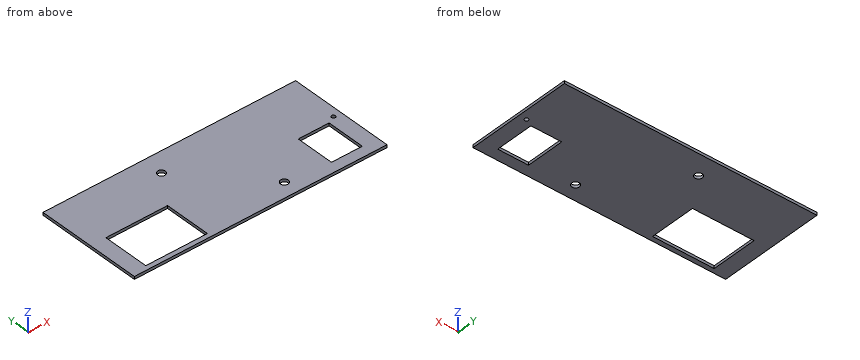
```python
from build123d import *

# Parameters (mm, degrees)
SKETCH_W      = 164
SKETCH_H      = 68.8
PAD_DEPTH     = 1.8
SKETCH001_R   = 2.5
SKETCH001_R_2 = 1.25
SKETCH001_W   = 40
SKETCH001_H   = 30
SKETCH001_W_2 = 20
SKETCH001_H_2 = 25
POCKET_DEPTH  = 5


with BuildPart() as part:
    # Sketch → Pad (new body)
    with BuildSketch(Plane.XY):
        with Locations((82, 34.4)):
            Rectangle(SKETCH_W, SKETCH_H)
    extrude(amount=PAD_DEPTH)

    # Sketch001 (on Face6 of Pad) → Pocket (cut)
    with BuildSketch(Plane.XY.offset(1.8)):
        with Locations((65, 55)):
            Circle(SKETCH001_R)
        with Locations((106, 10)):
            Circle(SKETCH001_R)
        with Locations((159, 34.5)):
            Circle(SKETCH001_R_2)
        with Locations((30, 18)):
            Rectangle(SKETCH001_W, SKETCH001_H)
        with Locations((144, 19.5)):
            Rectangle(SKETCH001_W_2, SKETCH001_H_2)
    extrude(amount=-POCKET_DEPTH, mode=Mode.SUBTRACT)


solid = part.part
```
Work out the finished part from the listing and answer in its coordinate system (mm). Give positions to 0.01 mm unless a question says otherwise; leave off trailing zeros. Order: outer loops, then holes, each group sorted by start corner. A loop starts at its lowest first (then second) coordinate and runs counter-clockwise, first axis right, second up.
1. Section C-C, the plane y = 55 is taken. Determine the outline of the cut face in (x, z).
Result sheet:
outline: (0, 0) - (62.5, 0) - (62.5, 1.8) - (0, 1.8) - close; (67.5, 0) - (164, 0) - (164, 1.8) - (67.5, 1.8) - close
2. Section B-B, the plane x = 142 is taken. Determine the outline of the cut face in (y, z), and give its area (3 significant figures).
Result sheet:
outline: (0, 0) - (7, 0) - (7, 1.8) - (0, 1.8) - close; (32, 0) - (68.8, 0) - (68.8, 1.8) - (32, 1.8) - close
area: 78.8 mm2
3. Section D-D, the plane z = 0.4 is taken. Determine the outline of the cut face in (x, y), and give its area (3 significant figures).
Result sheet:
outline: (0, 0) - (164, 0) - (164, 68.8) - (0, 68.8) - close; hole (10, 3) - (50, 3) - (50, 33) - (10, 33) - close; hole circle Ø5 at (65, 55); hole circle Ø5 at (106, 10); hole (134, 7) - (154, 7) - (154, 32) - (134, 32) - close; hole circle Ø2.5 at (159, 34.5)
area: 9,540 mm2
4. Section A-A, the plane y = 10 is taken. Determine the outline of the cut face in (x, z).
Result sheet:
outline: (0, 0) - (10, 0) - (10, 1.8) - (0, 1.8) - close; (50, 0) - (103.5, 0) - (103.5, 1.8) - (50, 1.8) - close; (108.5, 0) - (134, 0) - (134, 1.8) - (108.5, 1.8) - close; (154, 0) - (164, 0) - (164, 1.8) - (154, 1.8) - close
5. Straight lines are drawn through the part: L1, parallel to X at y = 28.5, z = 0.65; L2, parallel to Y at x = 106, z = 0.4; L3, parallel to Y at x = 159, z = 1.25. For each, find the intervals that lie inside material, in ascending order.
Result sheet:
L1: x = 0 to 10, 50 to 134, 154 to 164
L2: y = 0 to 7.5, 12.5 to 68.8
L3: y = 0 to 33.25, 35.75 to 68.8
